Geometry check sheet. Reference: the model listing, model coordinates, mm. Round coordinates to 2 decimals unless told otherwise and drop trailing zeros. Use one line per item in the form item = value.
Autodesk Inventor part; units mm, degrees
ref_plane "Arbeitsebene1" through (-76, 99, 0) normal (0, -1, 0) x (1, 0, 0)
ref_plane "YZ Plane" through (0, 0, 0) normal (1, 0, 0) x (0, 1, 0)
ref_plane "XZ Plane" through (0, 0, 0) normal (0, 1, 0) x (-1, 0, 0)
sketch "Skizze3" plane through (0, 0, 0) normal (0, 0, 1) x (1, 0, 0)
  line L0 (0, 0) -> (-76, 0)
  line L1 (-76, 0) -> (-76, 198)
  line L2 (-76, 198) -> (0, 198)
  line L3 (0, 198) -> (0, 0)
  point P0 (-13, 161)
  point P1 (-13, 147)
  point P2 (-71.81, 154)
  point P3 (-60, 144)
  dimension "d4" = 198
  dimension "d5" = 76
  dimension "d9" = 37
  dimension "d10" = 51
  dimension "d11" = 13
  dimension "d12" = 13
  dimension "d13" = 71.81
  dimension "d14" = 44
  dimension "d15" = 60
  dimension "d16" = 54
extrude "Extrusion3" add sketch "Skizze3" along normal blind 5
fillet "Rundung1" radius 2 4 edges at (0, 198, 2.5) (-76, 198, 2.5) (-76, 0, 2.5) (0, 0, 2.5)
ref_plane "Arbeitsebene1" through (-76, 99, 0) normal (0, -1, 0) x (1, 0, 0)
hole "Bohrung1" at (-13, 161, 0) at (-13, 147, 0) at (-60, 144, 0) direction (0, 0, 1) diameter 3.242 end through all
hole "Bohrung2" at (-71.81, 154, 0) direction (0, 0, 1) diameter 1.567 depth 4.2 tip angle 118 countersink diameter 4.5 countersink angle 90
mirror "Spiegeln1" about plane through (-76, 99, 0) normal (0, -1, 0) of "Bohrung2", "Bohrung1"
properties part number "BT703_trajan20_21" material "Acryl"
1. Material ranges on line 1 along Y through (x, z) = (-60, 2.4); line 2 along X through (y, z) = (161, 3.6); line 3 along Y through (x, z) = (-13, 1.1), recorded low to high.
Return value:
line_1 = 0 to 52.38, 55.62 to 142.38, 145.62 to 198
line_2 = -76 to -14.62, -11.38 to 0
line_3 = 0 to 35.38, 38.62 to 49.38, 52.62 to 145.38, 148.62 to 159.38, 162.62 to 198
2. Gauge pin test, flat end, axial feed: pin 1 (1.3 mm diameter, centred on x = -71.81, y = 44, fed in from -Z). Record the tip position at first contact, or that the pin passes through.
Return value:
pin_1 = 4.28
3. Mould release check, pull along X, two halves, no side actions. Record for faces 1 (the flat face through (-37, 0, 2)), 2 (the cylindrical face through (-11.9, 38.19, 2.54)), 3 (the cylindrical face through (-13.621, 49.503, 2.535)), 4 (the flat face through (0, 100, 2)): released by +X, released by -X, zero draft, split by the parting line, or undercut.
Return value:
face_1 = zero draft
face_2 = undercut
face_3 = undercut
face_4 = released by +X
